The model under review builds one solid part; all positions refer to its coordinate system, in mm. A direction names the side the tool comes from. Round coordinates to 2 decimals unless told otherwise and drop trailing zeros. Loops run counter-clockwise (first coordinate to the right, second up) from the corner with the lowest first, then second, coordinate; pieces in that order, holes last. Notation, with made-up numbers: M -11,73 L 9,73 A35 cw 9,107 Z; hole C -1.5,-10 d7. An arc over 180 degrees is marked long. One line per question, with ' | ' between items.
from build123d import *

# Parameters (mm, degrees)
SKETCH2_W           = 150
SKETCH2_H           = 387
SKETCH2_R           = 2.6
BOSS_EXTRUDE1_DEPTH = 4
CUT_EXTRUDE1_DEPTH  = 10


with BuildPart() as part:
    # Sketch2 → Boss-Extrude1 (new body)
    with BuildSketch(Plane.XY.offset(30)):
        with Locations((-125, -183.5)):
            Rectangle(SKETCH2_W, SKETCH2_H)
        with Locations((-190, 0)):
            Circle(SKETCH2_R, mode=Mode.SUBTRACT)
        with Locations((-60, 0)):
            Circle(SKETCH2_R, mode=Mode.SUBTRACT)
        with Locations((-125, 0)):
            Circle(SKETCH2_R, mode=Mode.SUBTRACT)
        with Locations((-60, -367)):
            Circle(SKETCH2_R, mode=Mode.SUBTRACT)
        with Locations((-125, -367)):
            Circle(SKETCH2_R, mode=Mode.SUBTRACT)
        with Locations((-190, -367)):
            Circle(SKETCH2_R, mode=Mode.SUBTRACT)
    extrude(amount=BOSS_EXTRUDE1_DEPTH)

    # Sketch3 → Cut-Extrude1 (cut)
    with BuildSketch(Plane.XY.offset(34)):
        with BuildLine():
            Line((-163.151021772, -10), (-86.848978228, -10))
            ThreePointArc((-86.848978228, -10), (-82.810612321, -12.051847901), (-82.086691458, -16.523359681))
            Line((-82.086691458, -16.523359681), (-120.23771323, -135.790075557))
            ThreePointArc((-120.23771323, -135.790075557), (-125, -139.266715876), (-129.76228677, -135.790075557))
            Line((-129.76228677, -135.790075557), (-167.913308542, -16.523359681))
            ThreePointArc((-167.913308542, -16.523359681), (-167.189387679, -12.051847901), (-163.151021772, -10))
        make_face()
        with BuildLine():
            Line((-180, -76.424605697), (-180, -290.575394303))
            ThreePointArc((-180, -290.575394303), (-175.770897577, -295.515608562), (-170.23771323, -292.098753984))
            Line((-170.23771323, -292.098753984), (-135.986449838, -185.023359681))
            ThreePointArc((-135.986449838, -185.023359681), (-135.748736609, -183.5), (-135.986449838, -181.976640319))
            Line((-135.986449838, -181.976640319), (-170.23771323, -74.901246016))
            ThreePointArc((-170.23771323, -74.901246016), (-175.770897577, -71.484391438), (-180, -76.424605697))
        make_face()
        with BuildLine():
            Line((-163.151021772, -357), (-86.848978228, -357))
            ThreePointArc((-86.848978228, -357), (-82.810612321, -354.948152099), (-82.086691458, -350.476640319))
            Line((-82.086691458, -350.476640319), (-120.23771323, -231.209924443))
            ThreePointArc((-120.23771323, -231.209924443), (-125, -227.733284124), (-129.76228677, -231.209924443))
            Line((-129.76228677, -231.209924443), (-167.913308542, -350.476640319))
            ThreePointArc((-167.913308542, -350.476640319), (-167.189387679, -354.948152099), (-163.151021772, -357))
        make_face()
        with BuildLine():
            Line((-70, -76.424605697), (-70, -290.575394303))
            ThreePointArc((-70, -290.575394303), (-74.229102423, -295.515608562), (-79.76228677, -292.098753984))
            Line((-79.76228677, -292.098753984), (-114.013550162, -185.023359681))
            ThreePointArc((-114.013550162, -185.023359681), (-114.251263391, -183.5), (-114.013550162, -181.976640319))
            Line((-114.013550162, -181.976640319), (-79.76228677, -74.901246016))
            ThreePointArc((-79.76228677, -74.901246016), (-74.229102423, -71.484391438), (-70, -76.424605697))
        make_face()
    extrude(amount=-CUT_EXTRUDE1_DEPTH, mode=Mode.SUBTRACT)


solid = part.part
1) Add section B-B on z = 32.05. State how many separate pieces and enclosed holes the cut face has, then the cut area to 3 significant figures.
Output values:
separate pieces: 1 | enclosed holes: 10 | area: 33,500 mm²
2) Mouldability with a two-part tool opening along X and no side actions: class faces 3 (the flat face through (-126, -181, 34)), 4 (the flat face through (-96.65, -239.31, 32.03)), 5 (the flat face through (-100.895, -75.322, 32.028)) as +X half, -X half, draft (parallel to the pull), parting line (faces both ways), or undercut.
Output values:
face 3: draft | face 4: undercut | face 5: undercut
3) Machinability: for faces 1 (the flat face through (-97.13, -129.19, 32.03)), 2 (the flat face through (-126, -181, 30)), which of the approach directions +Z, -Z, +X, -X, +Y, -Y give a long, thin tool a straight path to every point of the face, cutting with its end or side? Answer none if there is none.
Output values:
face 1: +Z, -Z | face 2: -Z, +X, -X, +Y, -Y
4) For line 1 (Y direction, x = -125, z = 32.6); line 2 (X direction, y = -367, z = 32); line 3 (X direction, y = -184, z = 31.75), list the stretches that pass through material, from the lowest coordinate up.
Output values:
line 1: y = -377 to -369.6, -364.4 to -357, -227.73 to -139.27, -10 to -2.6, 2.6 to 10 | line 2: x = -200 to -192.6, -187.4 to -127.6, -122.4 to -62.6, -57.4 to -50 | line 3: x = -200 to -180, -135.77 to -114.23, -70 to -50
5) Add section A-A on x = -176.5. State the section outline as (y, z) points, then the cut area to 3 significant figures.
Output values:
outline: M -377,30 L -295.35,30 L -295.35,34 L -377,34 Z; M -71.65,30 L 10,30 L 10,34 L -71.65,34 Z | area: 653 mm²
